from build123d import *

# Parameters (mm, degrees)
SKETCH1_W           = 55.88
SKETCH1_H           = 114.3
BOSS_EXTRUDE1_DEPTH = 8.3
SKETCH2_R           = 3.1
BOSS_EXTRUDE2_DEPTH = 12.7
LPATTERN1_COUNT     = 4
LPATTERN1_PITCH     = 28.575


with BuildPart() as part:
    # Sketch1 → Boss-Extrude1 (new body)
    with BuildSketch(Plane(origin=(0, 0, 0), x_dir=(0, 0, -1), z_dir=(1, 0, 0))):
        Rectangle(SKETCH1_W, SKETCH1_H)
    extrude(amount=BOSS_EXTRUDE1_DEPTH)

    # Sketch2 → Boss-Extrude2 (add)
    with BuildSketch(Plane.XY.offset(27.94)):
        with Locations(Location((4.15, -42.8625, 0), (0, 0, 90))):  # turned: the seam where the file's is
            Circle(SKETCH2_R)
    boss_extrude2 = extrude(amount=BOSS_EXTRUDE2_DEPTH)

    # LPattern1: Boss-Extrude2 ×4
    with Locations(*[(0, i * LPATTERN1_PITCH, 0) for i in range(1, LPATTERN1_COUNT)]):
        add(boss_extrude2)


solid = part.part
Geometry: final body of the model. Coordinates: model frame, mm. A direction names the side the tool comes from. Coordinates: 2 decimals unless noted, no trailing zeros. Loops run counter-clockwise (first coordinate to the right, second up) from the corner with the lowest first, then second, coordinate; pieces in that order, holes last. Notation, with made-up numbers: M 78,29 L 122,29 A23 ccw 122,66 Z; hole C 41.25,17.25 d6. An arc over 180 degrees is marked long. One line per item, written item: value. Start each with the question number.
1) Draft query along Y for faces 3 (the flat face through (4, -1, -27.94)), 4 (the flat face through (4, 57.15, 0)), 5 (the flat face through (4, -57.15, 0)), 6 (the cylindrical face through (5.34, -40, 34.2)). Return one class per face: released by +Y, released by -Y, zero draft, split by the parting line, or undercut.
2) Pin query (flat end, axial travel): P1, Ø3, axis at x = 1.5, z = 34, coming from the -Y side. Return the tip coordinate at first contact, or that it passes through.
3) Reachability of faces 1 (the flat face through (4, -14, 40.64)), 2 (the cylindrical face through (5.34, 17.15, 34.2)) from +Z, -Z, +X, -X, +Y, -Y: full face, straight path, thin tool, end or side. Return the list, or none.
4) Cut plane B-B (z = 34). Return loops of the section in (x, y), then the cut area to 3 significant figures.
5) Cut plane A-A (x = 4.15). Return loops of the section in (y, z), then the cut area to 3 significant figures.
6) Material intervals for L1, parallel to Z at x = 7.75, y = 35; L2, parallel to Y at x = 6.5, z = 34.5, sorted ascending. Write a range as from..to.
7) Cut plane C-C (y = -30). Return loops of the section in (x, z).
Evaluation:
1. face 3: zero draft
1. face 4: released by +Y
1. face 5: released by -Y
1. face 6: undercut
2. P1: y = -45.74
3. face 1: +Z, +X, -X, +Y, -Y
3. face 2: +Z
4. outline: C 4.15,-42.86 d6.2; C 4.15,-14.29 d6.2; C 4.15,14.29 d6.2; C 4.15,42.86 d6.2
4. area: 121 mm^2
5. outline: M -57.15,-27.94 L 57.15,-27.94 L 57.15,27.94 L 45.96,27.94 L 45.96,40.64 L 39.76,40.64 L 39.76,27.94 L 17.39,27.94 L 17.39,40.64 L 11.19,40.64 L 11.19,27.94 L -11.19,27.94 L -11.19,40.64 L -17.39,40.64 L -17.39,27.94 L -39.76,27.94 L -39.76,40.64 L -45.96,40.64 L -45.96,27.94 L -57.15,27.94 Z
5. area: 6,700 mm^2
6. L1: -27.94..27.94
6. L2: -44.88..-40.84, -16.31..-12.27, 12.27..16.31, 40.84..44.88
7. outline: M 0,-27.94 L 8.3,-27.94 L 8.3,27.94 L 0,27.94 Z
